Geometry: see drawing. Coordinates: mm, zero at the bounding-box minimum. A direction names the side the tool comes from. Coordinates: 2 decimals unless noted, no trailing zeros. Order: outer loops, then holes, each group sorted by start corner. A loop starts at its lowest first (then second) coordinate and runs counter-clockwise, first axis right, second up. Notation, with made-up numbers: M 73.25,12 L 100.25,12 A28 cw 100.25,46 Z; hole C -24,76.25 d7. An arc over 180 degrees is marked long. Answer in a Markdown table with one row per item.
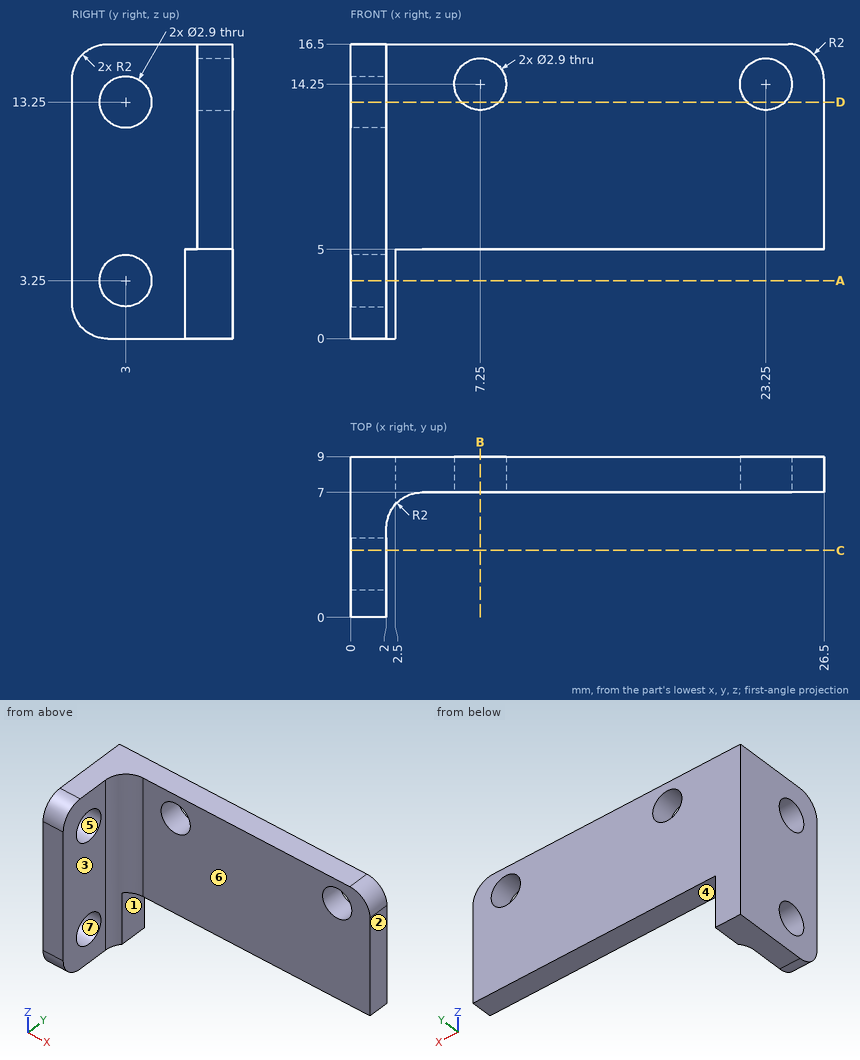
1) Reachability of the marked faces 1, 2 and 3 from +Z, -Z, +X, -X, +Y, -Y: full face, straight path, thin tool, end or side. Return the list, or none.
Resolved:
| item | result |
|---|---|
| face 1 | -Z, +X, +Y, -Y |
| face 2 | +Z, -Z, +X, +Y, -Y |
| face 3 | +Z, -Z, +X, -Y |
2) Cut plane A-A, the plane z = 3.25. Output: boundary loops of the cut face in (x, y), and give its area (3 significant figures).
Resolved:
| item | result |
|---|---|
| outline | M 0,0 L 2,0 L 2,1.55 L 0,1.55 Z; M 0,4.45 L 2,4.45 L 2,5 A2 cw 2.5,6.32 L 2.5,9 L 0,9 Z |
| area | 13.7 mm2 |
3) Material intervals for probe 1 along X at (y, z) = (8.35, 14.25); probe 2 along Y at (x, z) = (1.5, 13.25); probe 3 along Z at (x, y) = (23.25, 7.7), sorted ascending.
Resolved:
| item | result |
|---|---|
| probe 1 | x = 0 to 5.8, 8.7 to 21.8, 24.7 to 26.5 |
| probe 2 | y = 0 to 1.55, 4.45 to 9 |
| probe 3 | z = 5 to 12.8, 15.7 to 16.5 |
4) Cut plane C-C, the plane y = 3.75. Output: boundary loops of the cut face in (x, z), and give its area (3 significant figures).
Resolved:
| item | result |
|---|---|
| outline | M 0,0 L 2,0 L 2,2.01 L 0,2.01 Z; M 0,4.49 L 2,4.49 L 2,12.01 L 0,12.01 Z; M 0,14.49 L 2,14.49 L 2,16.5 L 0,16.5 Z |
| area | 23.1 mm2 |
5) Contact query for flat-ended pins moving along their axis: pin 1 (1.5 mm diameter, centred on y = 6, z = 5.5, fed in from +X); pin 2 (3 mm diameter, centred on y = 3.5, z = 7.5, fed in from +X); pin 3 (9 mm diameter, centred on x = 15, z = 11, fed in from -Y); pin 4 (1.7 mm diameter, centred on x = 7.25, z = 14.25, fed in from +Y). Output: stop coordinate, or through.
Resolved:
| item | result |
|---|---|
| pin 1 | stops at x = 3.03 |
| pin 2 | stops at x = 2 |
| pin 3 | stops at y = 7 |
| pin 4 | passes through |
6) Mould query, pull axis Y, two halves, no side actions, for the marked faces 4, 5, 6 and 7. Classes: +Y half, -Y half, draft (parallel to the pull), parting line (faces both ways), or undercut.
Resolved:
| item | result |
|---|---|
| face 4 | draft |
| face 5 | undercut |
| face 6 | -Y half |
| face 7 | undercut |
7) Cut plane B-B, the plane x = 7.25. Output: boundary loops of the cut face in (y, z).
Resolved:
| item | result |
|---|---|
| outline | M 7,5 L 9,5 L 9,12.8 L 7,12.8 Z; M 7,15.7 L 9,15.7 L 9,16.5 L 7,16.5 Z |
8) Cut plane D-D, the plane z = 13.25. Output: boundary loops of the cut face in (x, y).
Resolved:
| item | result |
|---|---|
| outline | M 0,0 L 2,0 L 2,1.55 L 0,1.55 Z; M 0,4.45 L 2,4.45 L 2,5 A2 cw 4,7 L 6.2,7 L 6.2,9 L 0,9 Z; M 8.3,7 L 22.2,7 L 22.2,9 L 8.3,9 Z; M 24.3,7 L 26.5,7 L 26.5,9 L 24.3,9 Z |
